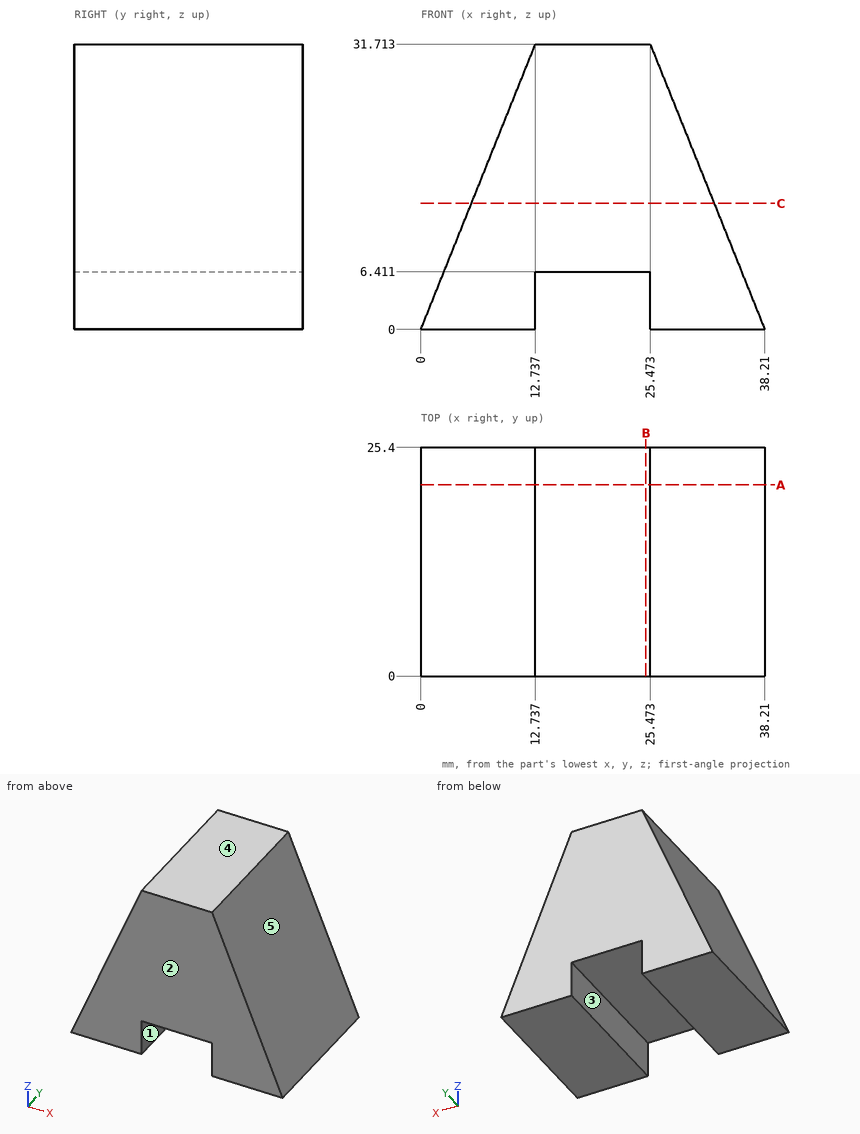
Job drawing, mm, ordinate dimensions from the low corner. One solid piece. A direction names the side the tool comes from. Give positions to 0.01 mm unless a question says otherwise; leave off trailing zeros. Loops run counter-clockwise (first coordinate to the right, second up) from the corner with the lowest first, then second, coordinate; pieces in that order, holes last. Notation, with made-up numbers: M 46,47.25 L 68,47.25 A29 ccw 68,81.25 Z; hole C -18.75,66.25 d4. An arc over 180 degrees is marked long. Return JSON: item names as keys, results as strings.
1) Drill centre lines: line 1 (Z direction, x = 14, y = 16.5); line 2 (X direction, y = 11.5, z = 1); line 3 (X direction, y = 18.75, z = 5.5). Where is each one in solid material? Low to high.
Calculated:
{"line 1": "z = 6.41 to 31.71", "line 2": "x = 0.4 to 12.74, 25.47 to 37.81", "line 3": "x = 2.21 to 12.74, 25.47 to 36"}
2) 3-axis set-ups, long thin cutter, end or side, ignore diameter. For the marked faces 1 and 2: which of +Z, -Z, +X, -X, +Y, -Y reach the whole face in a straight line?
Calculated:
{"face 1": "-Z, +Y, -Y", "face 2": "+Z, -Z, +X, -X, -Y"}
3) Pull direction X, two halves, no side cores. Call the marked faces 3, 4 and 5: released by +X, released by -X, zero draft, split by the parting line, or undercut.
Calculated:
{"face 3": "undercut", "face 4": "zero draft", "face 5": "released by +X"}
4) Saw through at A-A, the plane y = 21.25. List the corners of the cut face in (x, z), then the cut area to 3 significant figures.
Calculated:
{"outline": "M 0,0 L 12.74,0 L 12.74,6.41 L 25.47,6.41 L 25.47,0 L 38.21,0 L 25.47,31.71 L 12.74,31.71 Z", "area": "726 mm2"}
5) Saw through at B-B, the plane x = 25. List the corners of the cut face in (y, z), then the cut area to 3 significant figures.
Calculated:
{"outline": "M 0,6.41 L 25.4,6.41 L 25.4,31.71 L 0,31.71 Z", "area": "643 mm2"}
6) Flat gauge pins, fed straight in: pin 1 Ø5 at (y, z) = (8, 5) entering from -X; pin 2 Ø1 at (y, z) = (3, 6.5) entering from -X; pin 3 Ø5 at (y, z) = (5, 25.5) entering from -X. Where does each tip first touch, or does it go through?
Calculated:
{"pin 1": "stops at x = 1", "pin 2": "stops at x = 2.41", "pin 3": "stops at x = 9.24"}
7) Saw through at C-C, the plane z = 14. List the corners of the cut face in (x, y).
Calculated:
{"outline": "M 5.62,0 L 32.59,0 L 32.59,25.4 L 5.62,25.4 Z"}
